Geometry check sheet. Reference: the model listing, model coordinates, mm. Round coordinates to 2 decimals unless told otherwise and drop trailing zeros. Order: outer loops, then holes, each group sorted by start corner. A loop starts at its lowest first (then second) coordinate and runs counter-clockwise, first axis right, second up. Notation, with made-up numbers: (-22, -12.5) - (-5, -12.5) arc R15 ccw to (-5, 16.5) - close; hole circle Ø8 at (81.5, 67). An arc over 180 degrees is marked (long way). One line per question, with ' | ' between items. Start each with the question number.
Q1. Gauge pin test, flat ends, axial feed: P1, Ø1.5, axis at y = 5.5, z = 25, coming from the +X side; P2, Ø4, axis at y = 16, z = -1, coming from the -X side; P3, Ø4, axis at x = -9.5, y = 9.5, coming from the +Z side. Record the tip position at first contact, or that the pin passes through.
Q2. Material ranges on line 1 along X through (y, z) = (12.5, 0); line 2 along Z through (x, y) = (24.5, 8); line 3 along Z through (x, y) = (39, 10.25), recorded low to high.
Q3. Mould release check, pull along Z, two halves, no side actions. Record for faces 1 (the face through (-59.884, 9.888, 31.147)), 2 (the face through (-18.77, 9.86, -24.19)), 3 (the face through (-14, 20, -1)): +Z half, -Z half, draft (parallel to the pull), parting line (faces both ways), or undercut.
Q4. Sectioned sample at B-B, the plane y = 16. Give the number of separate pieces and of enclosed holes in the cut face, then the cut area to 3 significant figures.
Q5. Sectioned sample at A-A, the plane z = 0. Enter the section's corners in (x, y), then the cut area to 3 significant figures.
```python
from build123d import *

# Parameters (mm, degrees)
SKETCH1_R           = 67.5
BOSS_EXTRUDE1_DEPTH = 20
FILLET1_R           = 2
SKETCH2_R           = 7.5
CUT_EXTRUDE1_DEPTH  = 98.532046085
CUT_EXTRUDE2_DEPTH  = 98.532046085
CIRPATTERN1_COUNT   = 7
CIRPATTERN1_ANGLE   = 306


with BuildPart() as part:
    # Sketch1 → Boss-Extrude1 (new body)
    with BuildSketch(Plane(origin=(0, 0, 0), x_dir=(1, 0, 0), z_dir=(0, 1, 0))):
        with Locations(Location((0, 0, 0), (0, 0, 270))):
            Circle(SKETCH1_R)
    extrude(amount=BOSS_EXTRUDE1_DEPTH)

    # Fillet1
    fillet1_edges = [part.edges().sort_by_distance(p)[0] for p in [
        (0, 0, -67.5),
        (0, 20, -67.5),
    ]]
    fillet(fillet1_edges, radius=FILLET1_R)

    # Sketch2 → Cut-Extrude1 (cut, through all)
    with BuildSketch(Plane(origin=(0, 20, 0), x_dir=(1, 0, 0), z_dir=(0, 1, 0))):
        with Locations(Location((0, 0, 0), (0, 0, 270))):
            Circle(SKETCH2_R)
    extrude(amount=-CUT_EXTRUDE1_DEPTH, mode=Mode.SUBTRACT)

    # Sketch3 → Cut-Extrude2 (cut, through all)
    with BuildSketch(Plane.XZ):
        with BuildLine():
            Line((0, 30.617728898), (0, 55.617728898))
            ThreePointArc((0, 55.617728898), (13.100293951, 54.052882126), (25.463414591, 49.446398101))
            Line((25.463414591, 49.446398101), (14.017687169, 27.220392527))
            ThreePointArc((14.017687169, 27.220392527), (7.21175166, 29.756275991), (0, 30.617728898))
        make_face()
    cut_extrude2 = extrude(amount=-CUT_EXTRUDE2_DEPTH, mode=Mode.SUBTRACT)

    # CirPattern1: Cut-Extrude2 ×7 about axis
    cirpattern1_axis = Axis((0, 0, 0), (0, 1, 0))
    for i in range(1, CIRPATTERN1_COUNT):
        add(cut_extrude2.rotate(cirpattern1_axis, i * CIRPATTERN1_ANGLE / (CIRPATTERN1_COUNT - 1)), mode=Mode.SUBTRACT)


solid = part.part
```
Determined:
1) P1: stops at x = 62.99 | P2: stops at x = -67.5 | P3: stops at z = 67.08
2) line 1: x = -67.5 to -55.62, -30.62 to -7.5, 7.5 to 67.5 | line 2: z = -62.9 to -49.93, -48.08 to -20.02, -18.36 to 18.36, 19.84 to 47.58, 49.93 to 62.9 | line 3: z = -55.09 to -31.86, -8.29 to 8.11, 31.58 to 55.09
3) face 1: parting line | face 2: undercut | face 3: draft
4) separate pieces: 1 | enclosed holes: 8 | area: 10,500 mm2
5) outline: (-67.5, 2) arc R2 ccw to (-65.5, 0) - (-55.62, 0) - (-55.62, 20) - (-65.5, 20) arc R2 ccw to (-67.5, 18) - close; (-30.62, 0) - (-7.5, 0) - (-7.5, 20) - (-30.62, 20) - close; (7.5, 0) - (65.5, 0) arc R2 ccw to (67.5, 2) - (67.5, 18) arc R2 ccw to (65.5, 20) - (7.5, 20) - close | area: 1,900 mm2
